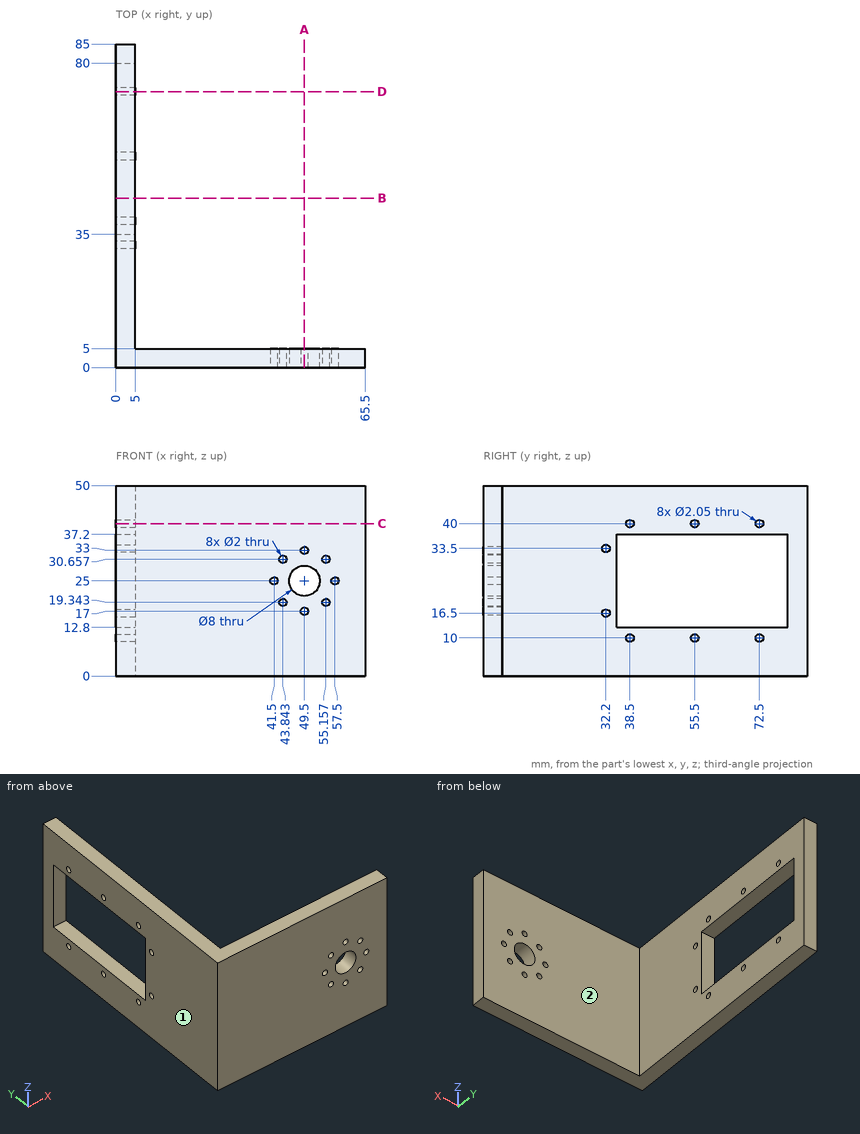
The figure shows three views and two pictorial views of one solid part (mm, origin at its lowest corner). Answer the questions. A direction names the side the tool comes from. Give positions to 0.01 mm unless a question says otherwise; leave off trailing zeros. Order: outer loops, then holes, each group sorted by start corner. A loop starts at its lowest first (then second) coordinate and runs counter-clockwise, first axis right, second up. Notation, with made-up numbers: (43.5, 35) -> (96.5, 35) arc R17 ccw to (96.5, 39) -> close; hole circle Ø10 at (-36.75, 32.5). An arc over 180 degrees is marked (long way). One line per item, written item: value.
1) Find section C-C, the plane z = 40. Determine the outline of the cut face in (x, y) (3 decimals), plus the area to 3 significant figures.
Reported:
outline: (0, 0) -> (65.5, 0) -> (65.5, 5) -> (5, 5) -> (5, 37.475) -> (0, 37.475) -> close; (0, 39.525) -> (5, 39.525) -> (5, 54.475) -> (0, 54.475) -> close; (0, 56.525) -> (5, 56.525) -> (5, 71.475) -> (0, 71.475) -> close; (0, 73.525) -> (5, 73.525) -> (5, 85) -> (0, 85) -> close
area: 697 mm^2
2) Find section A-A, the plane x = 49.5. Determine the outline of the cut face in (y, z), plus the area to 3 significant figures.
Reported:
outline: (0, 0) -> (5, 0) -> (5, 16) -> (0, 16) -> close; (0, 18) -> (5, 18) -> (5, 21) -> (0, 21) -> close; (0, 29) -> (5, 29) -> (5, 32) -> (0, 32) -> close; (0, 34) -> (5, 34) -> (5, 50) -> (0, 50) -> close
area: 190 mm^2
3) Flat-ended cylindrical pins translate along their axes: P1, Ø2.5, axis at x = 55.16, z = 19.34, coming from the +Y side; P2, Ø25, axis at y = 46.5, z = 36.5, coming from the +X side; P3, Ø1.2, axis at y = 38.5, z = 10, coming from the -X side. Find the tip coordinate at first contact, or state that the pin passes through.
Reported:
P1: stops at y = 5
P2: stops at x = 5
P3: passes through
4) Find section B-B, the plane y = 44.5. Determine the outline of the cut face in (x, z), plus the area to 3 significant figures.
Reported:
outline: (0, 0) -> (5, 0) -> (5, 12.8) -> (0, 12.8) -> close; (0, 37.2) -> (5, 37.2) -> (5, 50) -> (0, 50) -> close
area: 128 mm^2
5) Find the intervals of material crossed by line 1 (Y direction, x = 1, z = 10) (3 decimals); line 2 (Y direction, x = 1.2, z = 33.5) (3 decimals); line 3 (X direction, y = 3, z = 33), in increasing order.
Reported:
line 1: y = 0 to 37.475, 39.525 to 54.475, 56.525 to 71.475, 73.525 to 85
line 2: y = 0 to 31.175, 33.225 to 35, 80 to 85
line 3: x = 0 to 48.5, 50.5 to 65.5
6) A tool of negligible diameter and unlimited length cuts with its end or side. For the marked faces 1 and 2, from which of +Z, -Z, +X, -X, +Y, -Y can it reach the whole face along a straight path? Write none if from no direction.
Reported:
face 1: +Z, -Z, -X, +Y, -Y
face 2: +Z, -Z, +X, +Y
7) Find section D-D, the plane y = 72.5. Determine the outline of the cut face in (x, z) (3 decimals), plus the area to 4 significant figures.
Reported:
outline: (0, 0) -> (5, 0) -> (5, 8.975) -> (0, 8.975) -> close; (0, 11.025) -> (5, 11.025) -> (5, 12.8) -> (0, 12.8) -> close; (0, 37.2) -> (5, 37.2) -> (5, 38.975) -> (0, 38.975) -> close; (0, 41.025) -> (5, 41.025) -> (5, 50) -> (0, 50) -> close
area: 107.5 mm^2
